from build123d import *

# Parameters (mm, degrees)
F1_DEPTH = 58.928
F2_R     = 16.356515
F3_DEPTH = 79.502
F4_R     = 5.399917
F5_DEPTH = 98.044
F6_R     = 5.056805
F6_R_2   = 5.705972
F7_DEPTH = 93.726


with BuildPart() as f1:
    # F0 (on Top) → F1 (new body)
    with BuildSketch(Plane.XY):
        with BuildLine():
            Line((45.224381, -25.4), (45.224381, 25.4))
            Line((45.224381, 25.4), (22.640265, 25.4))
            ThreePointArc((22.640265, 25.4), (0, 48.040265), (-22.640265, 25.4))
            Line((-22.640265, 25.4), (-45.224381, 25.4))
            Line((-45.224381, 25.4), (-45.224381, -25.4))
            Line((-45.224381, -25.4), (45.224381, -25.4))
        make_face()
    extrude(amount=F1_DEPTH)

    # F2 (on face) → F3 (cut)
    with BuildSketch(Plane.XY.offset(58.928)):
        with Locations((0, 25.4)):
            Circle(F2_R)
    extrude(amount=-F3_DEPTH, mode=Mode.SUBTRACT)

    # F4 (on face) → F5 (cut)
    with BuildSketch(Plane(origin=(0, 25.4, 0), x_dir=(-1, 0, 0), z_dir=(0, 1, 0))):
        with Locations((33.932323, 12.529076)):
            Circle(F4_R)
        with Locations((34.354472, 46.398924)):
            Circle(F4_R)
    extrude(amount=-F5_DEPTH, mode=Mode.SUBTRACT)

    # F6 (on face) → F7 (cut)
    with BuildSketch(Plane(origin=(0, 25.4, 0), x_dir=(-1, 0, 0), z_dir=(0, 1, 0))):
        with Locations((-33.932323, 10.271089)):
            Circle(F6_R)
        with Locations((-33.932323, 45.897149)):
            Circle(F6_R_2)
    extrude(amount=-F7_DEPTH, mode=Mode.SUBTRACT)


solid = f1.part
The model under review builds one solid part; all positions refer to its coordinate system, in mm. A direction names the side the tool comes from. Give positions to 0.01 mm unless a question says otherwise; leave off trailing zeros. Write each loop counter-clockwise with the first axis right and the second up, starting at its lowest first coordinate (ties: lowest second). Pieces come first, ordered by that corner, then holes.
1. Add section B-B, the plane z = 48. Write out the cut boundary in (x, y), plus the area to 3 significant figures.
2. Add section C-C, the plane x = 0. Write out the cut boundary in (y, z), plus the area to 3 significant figures.
3. Add section A-A, the plane y = 21. Write out the cut boundary in (x, z), plus the area to 3 significant figures.
4. Wall thickness on L1, parallel to Y at x = 0, z = 15.5; L2, parallel to X at y = 25, z = 20; L3, parallel to Z at x = 30, y = 4: over which ranges is each line inside the solid? List them lowest first.
5. Draft analysis for pull direction Z (two halves, no side actions). For faces 4 (the flat face through (-1, 4, 58.928)), 5 (the cylindrical face through (35.169, 0.356, 40.327)), 6 (the flat face through (-45.224, 0, 29)), state which applies: +Z half, -Z half, draft (parallel to the pull), parting line (faces both ways), or undercut.
6. Add section D-D, the plane z = 36. Write out the cut boundary in (x, y), plus the area to 3 significant figures.
7. Tool access review of faces 1 (the flat face through (-34, 25.4, 29)), 2 (the cylindrical face through (-33.18, 0.36, 41.13)), 3 (the flat face through (34, 25.4, 29)): name each direction out of +Z, -Z, +X, -X, +Y, -Y from which nothing blocks a thin tool from reaching the whole face with its end or side.
8. For P1, Ø8, axis at x = 33.93, z = 10.27, coming from the -Y side; P2, Ø11.5, axis at x = -39, z = 18, coming from the +Y side; P3, Ø10, axis at x = 12.5, y = 20.5, coming from the -Z side, all flat-tipped, find the tip position at first contact; note any pin that passes through.
Worked answers:
1. outline: (-45.22, -25.4) - (-39.51, -25.4) - (-39.51, 25.4) - (-45.22, 25.4) - close; (-29.2, -25.4) - (28.63, -25.4) - (28.63, 25.4) - (22.64, 25.4) arc R22.64 ccw to (-22.64, 25.4) - (-29.2, 25.4) - close; (39.24, -25.4) - (45.22, -25.4) - (45.22, 25.4) - (39.24, 25.4) - close; hole circle Ø32.71 at (0, 25.4)
1. area: 3,500 mm2
2. outline: (-25.4, 0) - (9.04, 0) - (9.04, 58.93) - (-25.4, 58.93) - close; (41.76, 0) - (48.04, 0) - (48.04, 58.93) - (41.76, 58.93) - close
2. area: 2,400 mm2
3. outline: (-45.22, 0) - (-15.75, 0) - (-15.75, 58.93) - (-45.22, 58.93) - close; (15.75, 0) - (45.22, 0) - (45.22, 58.93) - (15.75, 58.93) - close; hole circle Ø10.8 at (-34.35, 46.4); hole circle Ø10.8 at (-33.93, 12.53); hole circle Ø11.41 at (33.93, 45.9); hole circle Ø10.11 at (33.93, 10.27)
3. area: 3,110 mm2
4. L1: y = -25.4 to 9.04, 41.76 to 48.04
4. L2: x = -45.22 to -16.35, 16.35 to 45.22
4. L3: z = 0 to 7.09, 13.45 to 41.76, 50.03 to 58.93
5. face 4: +Z half
5. face 5: undercut
5. face 6: draft
6. outline: (-45.22, -25.4) - (45.22, -25.4) - (45.22, 25.4) - (22.64, 25.4) arc R22.64 ccw to (-22.64, 25.4) - (-45.22, 25.4) - close; hole circle Ø32.71 at (0, 25.4)
6. area: 4,560 mm2
7. face 1: +Z, -Z, -X, +Y
7. face 2: +Y, -Y
7. face 3: +Z, -Z, +X, +Y
8. P1: passes through
8. P2: stops at y = 25.4
8. P3: stops at z = 0
